```python
from build123d import *

# Parameters (mm, degrees)
BOSS_EXTRUDE1_DEPTH = 3
SKETCH2_W           = 20
SKETCH2_H           = 15
CUT_EXTRUDE2_DEPTH  = 10


with BuildPart() as part:
    # Sketch1 → Boss-Extrude1 (new body)
    with BuildSketch(Plane.XY):
        Polygon((41.712301942, -43.626199709), (41.712301942, -55.563699709), (44.712301942, -55.563699709), (44.712301942, -74.688699709), (41.712301942, -74.688699709), (41.712301942, -86.626199709), (65.149801942, -86.626199709), (65.149801942, -83.626199709), (84.274801942, -83.626199709), (84.274801942, -86.626199709), (103.399801942, -86.626199709), (107.712301942, -86.626199709), (107.712301942, -74.688699709), (104.712301942, -74.688699709), (104.712301942, -55.563699709), (107.712301942, -55.563699709), (107.712301942, -43.626199709), align=None)
    extrude(amount=BOSS_EXTRUDE1_DEPTH)

    # Sketch2 → Cut-Extrude2 (cut)
    with BuildSketch(Plane.XY.offset(3)):
        with Locations((76.712301942, -65.632728749)):
            Rectangle(SKETCH2_W, SKETCH2_H)
    extrude(amount=-CUT_EXTRUDE2_DEPTH, mode=Mode.SUBTRACT)


solid = part.part
```
Verification items for the finished model (mm, model axes). A direction names the side the tool comes from. Give positions to 0.01 mm unless a question says otherwise; leave off trailing zeros. Write each loop counter-clockwise with the first axis right and the second up, starting at its lowest first coordinate (ties: lowest second). Pieces come first, ordered by that corner, then holes. Notation, with made-up numbers: M 14.25,69.5 L 56.25,69.5 A7 ccw 56.25,77.5 Z; hole C 69.5,31 d10. An arc over 180 degrees is marked long. One line per question, with ' | ' between items.
1) Set-up check for faces 1 (the flat face through (77, -58.133, 2)), 2 (the flat face through (106, -55.564, 1)), 3 (the flat face through (43, -74.689, 1)), 4 (the flat face through (65.15, -85, 1)): record each of +Z, -Z, +X, -X, +Y, -Y from which the full face is reachable in a straight line by a thin tool's end or side.
Result:
face 1: +Z, -Z | face 2: +Z, -Z, +X | face 3: +Z, -Z, -X | face 4: +Z, -Z, -Y
2) Section check C-C on z = 0.6. Enter the section's corners in (x, y), plus the area to 3 significant figures.
Result:
outline: M 41.71,-86.63 L 65.15,-86.63 L 65.15,-83.63 L 84.27,-83.63 L 84.27,-86.63 L 107.71,-86.63 L 107.71,-74.69 L 104.71,-74.69 L 104.71,-55.56 L 107.71,-55.56 L 107.71,-43.63 L 41.71,-43.63 L 41.71,-55.56 L 44.71,-55.56 L 44.71,-74.69 L 41.71,-74.69 Z; hole M 66.71,-73.13 L 86.71,-73.13 L 86.71,-58.13 L 66.71,-58.13 Z | area: 2,370 mm2
3) Thickness scan on line 1 along X through (y, z) = (-61, 2.4); line 2 along Y through (x, z) = (67, 1.6); line 3 along Y through (x, z) = (105.5, 0.85). Record the ranges inside material, lowest first. Write a range as [from, to].
Result:
line 1: x = [44.71, 66.71], [86.71, 104.71] | line 2: y = [-83.63, -73.13], [-58.13, -43.63] | line 3: y = [-86.63, -74.69], [-55.56, -43.63]
4) Gauge pin test, flat ends, axial feed: pin 1 Ø1.5 at (x, z) = (77, 2) entering from -Y; pin 2 Ø1.5 at (y, z) = (-66.5, 2) entering from -X; pin 3 Ø2 at (x, y) = (91.5, -70.5) entering from -Z; pin 4 Ø1.5 at (y, z) = (-66, 2) entering from +X. Record the tip position at first contact, or that the pin passes through.
Result:
pin 1: stops at y = -83.63 | pin 2: stops at x = 44.71 | pin 3: stops at z = 0 | pin 4: stops at x = 104.71
5) Mould release check, pull along Y, two halves, no side actions. Record for faces 5 (the flat face through (53, -86.626, 1)), 6 (the flat face through (86.712, -66, 2)), 7 (the flat face through (75, -43.626, 1)), 8 (the flat face through (41.712, -81, 1)): released by +Y, released by -Y, zero draft, split by the parting line, or undercut.
Result:
face 5: released by -Y | face 6: undercut | face 7: released by +Y | face 8: zero draft
6) Section check A-A on x = 81. Enter the section's corners in (y, z).
Result:
outline: M -83.63,0 L -73.13,0 L -73.13,3 L -83.63,3 Z; M -58.13,0 L -43.63,0 L -43.63,3 L -58.13,3 Z
7) Section check B-B on y = -69. Enter the section's corners in (x, z).
Result:
outline: M 44.71,0 L 66.71,0 L 66.71,3 L 44.71,3 Z; M 86.71,0 L 104.71,0 L 104.71,3 L 86.71,3 Z
